Source: three-view drawing plus pictorial views. Frame: mm from the lowest corner of the part. A direction names the side the tool comes from. Give positions to 0.01 mm unless a question says otherwise; leave off trailing zeros. Write each loop counter-clockwise with the first axis right and the second up, starting at its lowest first coordinate (ties: lowest second). Pieces come first, ordered by that corner, then holes. Notation, with made-up numbers: (-14.5, 84.25) -> (4.5, 84.25) arc R11 cw to (4.5, 102.25) -> close; hole circle Ø11 at (-33, 10). An arc over 180 degrees is marked (long way). Answer in a Markdown table with one row per item. Add a question column.
Item 1: Draft query along X for the marked faces 1, 2 and 3. Return one class per face: +X half, -X half, draft (parallel to the pull), parting line (faces both ways), or undercut.
Item 2: First-contact query: P1, Ø1.5, axis at x = 33.5, z = 19, coming from the -Y side; P2, Ø5, axis at x = 7.5, z = 22.5, coming from the +Y side; P3, Ø6, axis at x = 61.5, z = 14, coming from the +Y side; P4, Ø12, axis at x = 37, z = 10.5, coming from the -Y side. Flat tips, straight axial feed; report the tip coordinate or a pass-through.
Item 3: Section query A-A on z = 22.5. Output: boundary loops of the cut face in (x, y).
Item 4: Access query for the marked faces 4, 5, 6, 7 and 8. Directions: +Z, -Z, +X, -X, +Y, -Y. A direction counts if a zero-diameter tool reaches every point of the face in a straight line with its end or side. Return the directions, or none.
Item 5: Material intervals for probe 1 along Z at (x, y) = (102.5, 3.65); probe 2 along X at (y, z) = (10.5, 27); probe 3 along X at (y, z) = (27, 14), sorted ascending. Write a range as from..to.
Item 6: Section query D-D on z = 27.5. Output: boundary loops of the cut face in (x, y).
Item 7: Section query C-C on y = 41. Output: boundary loops of the cut face in (x, z).
Item 8: Section query B-B on x = 102.5. Output: boundary loops of the cut face in (y, z).
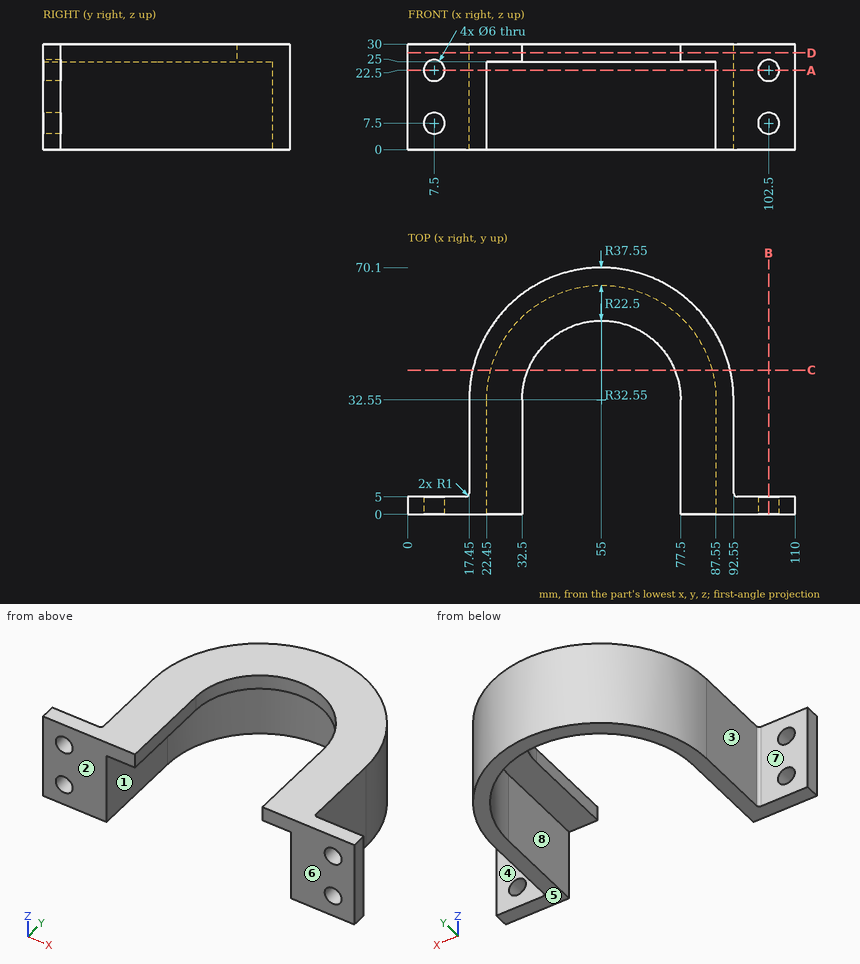
Findings below:
| question | item | result |
|---|---|---|
| 1 | face 1 | undercut |
| 1 | face 2 | draft |
| 1 | face 3 | -X half |
| 2 | P1 | stops at y = 56.31 |
| 2 | P2 | passes through |
| 2 | P3 | stops at y = 69.94 |
| 2 | P4 | stops at y = 54.54 |
| 3 | outline | (0, 0) -> (4.5, 0) -> (4.5, 5) -> (0, 5) -> close; (10.5, 0) -> (22.45, 0) -> (22.45, 32.55) arc R32.55 cw to (87.55, 32.55) -> (87.55, 0) -> (99.5, 0) -> (99.5, 5) -> (93.55, 5) arc R1 cw to (92.55, 6) -> (92.55, 32.55) arc R37.55 ccw to (17.45, 32.55) -> (17.45, 6) arc R1 cw to (16.45, 5) -> (10.5, 5) -> close; (105.5, 0) -> (110, 0) -> (110, 5) -> (105.5, 5) -> close |
| 4 | face 4 | +Z, -Z, +X, +Y |
| 4 | face 5 | -Z, +X, -X, +Y, -Y |
| 4 | face 6 | +Z, -Z, +X, -X, -Y |
| 4 | face 7 | +Z, -Z, -X, +Y |
| 4 | face 8 | -Z, -Y |
| 5 | probe 1 | z = 0..4.5, 10.5..19.5, 25.5..30 |
| 5 | probe 2 | x = 17.45..32.5, 77.5..92.55 |
| 5 | probe 3 | x = 17.45..22.45, 87.55..92.55 |
| 6 | outline | (0, 0) -> (32.5, 0) -> (32.5, 32.55) arc R22.5 cw to (77.5, 32.55) -> (77.5, 0) -> (110, 0) -> (110, 5) -> (93.55, 5) arc R1 cw to (92.55, 6) -> (92.55, 32.55) arc R37.55 ccw to (17.45, 32.55) -> (17.45, 6) arc R1 cw to (16.45, 5) -> (0, 5) -> close |
| 7 | outline | (18.41, 0) -> (23.57, 0) -> (23.57, 25) -> (34.15, 25) -> (34.15, 30) -> (18.41, 30) -> close; (75.85, 25) -> (86.43, 25) -> (86.43, 0) -> (91.59, 0) -> (91.59, 30) -> (75.85, 30) -> close |
| 8 | outline | (0, 0) -> (5, 0) -> (5, 4.5) -> (0, 4.5) -> close; (0, 10.5) -> (5, 10.5) -> (5, 19.5) -> (0, 19.5) -> close; (0, 25.5) -> (5, 25.5) -> (5, 30) -> (0, 30) -> close |
